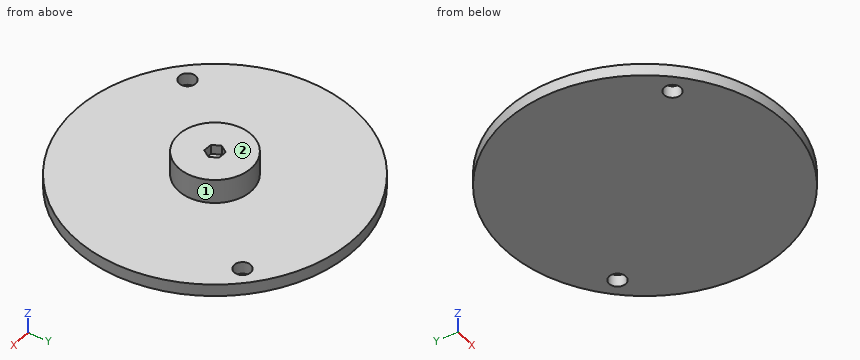
Autodesk Fusion 360 part; units mm, degrees
sketch "Sketch1" plane through (0, 0, 0) normal (0, 0, 1) x (1, 0, 0)
  circle A0 centre (0, 0) radius 18.2563
  line L0 (0, 0) -> (18.2563, 0) construction
  circle A1 centre (22.4506, 22.4506) radius 2.159
  circle A2 centre (-22.4506, -22.4506) radius 2.159
  circle A3 centre (0, 0) radius 9.525
  circle A4 centre (0, 0) radius 36.5125
  circle A5 centre (0, 0) radius 31.75
  line L1 (0, 0) -> (22.4506, 22.4506)
  line L2 (0, 0) -> (21.082, 0) construction
  line L3 (0, 0) -> (-22.4506, -22.4506)
  line L4 (0, 0) -> (21.082, 0) construction
  dimension "d1" = 36.5125
  dimension "d16" = 4.318
  dimension "d18" = 4.318
  dimension "d24" = 19.05
  dimension "d33" = 73.025
  dimension "d34" = 63.5
  dimension "d35" = 45
  dimension "d36" = 135
extrude "Extrude2" add sketch "Sketch1" along normal blind 3.175 contours A0 A3 L1 L3 | A0 A3 L1 L3 | A3 L1 L3 | A3 L1 L3
sketch "Sketch2" plane through (0, 0, 3.175) normal (0, 0, 1) x (-1, 0, 0)
  circle A0 centre (0, 0) radius 18.2563
  circle A1 centre (0, 0) radius 9.525
  dimension "d27" = 19.05
extrude "Extrude3" add sketch "Sketch2" along normal blind 6.35 contours A1
sketch "Sketch3" plane through (0, 0, 9.525) normal (0, 0, 1) x (-1, 0, 0)
  circle A0 centre (0, 0) radius 9.525
  line L0 (-1.2943, -1.9151) -> (1.0113, -2.0784)
  line L1 (1.0113, -2.0784) -> (2.3056, -0.1633)
  line L2 (2.3056, -0.1633) -> (1.2943, 1.9151)
  line L3 (1.2943, 1.9151) -> (-1.0113, 2.0784)
  line L4 (-1.0113, 2.0784) -> (-2.3056, 0.1633)
  line L5 (-2.3056, 0.1633) -> (-1.2943, -1.9151)
  dimension "d42" = 2.3114
extrude "Extrude7" add sketch "Sketch1" along normal blind 3.175 contours A0 A1 A2 A5 L1 L3 | A0 A1 A2 A5 L1 L3 | A4
extrude "Extrude8" cut sketch "Sketch3" against normal blind 2.3813 contours L0 L1 L2 L3 L4 L5
extrude "Extrude6" add sketch "Sketch1" along normal blind 3.175 contours A0 A1 A2 A5 L1 L3 | A0 A1 A2 A5 L1 L3 | A4
extrude "Extrude4" cut sketch "Sketch3" against normal blind 2.5 contours L0 L1 L2 L3 L4 L5
extrude "Extrude5" add sketch "Sketch1" along normal blind 3.175 contours A0 A1 A2 A5 L1 L3 | A0 A1 A2 A5 L1 L3 | A4
equation "d1 = ( 23 / 16 ) * 1 in"
equation "d45 = ( -3 / 32 ) * 1 in"
Source: CAD feature listing. Evaluate the final solid. Frame: model axes, mm. Face numbers are marked on the shaded views. A direction names the side the tool comes from. Round coordinates to 2 decimals unless told otherwise and drop trailing zeros. Order: outer loops, then holes, each group sorted by start corner. A loop starts at its lowest first (then second) coordinate and runs counter-clockwise, first axis right, second up. Notation, with made-up numbers: (31, 58.25) -> (48, 58.25) arc R24 ccw to (48, 78.25) -> close; hole circle Ø9 at (-31, 52). An arc over 180 degrees is marked (long way). One line per item, written item: value. Start each with the question number.
Q1. Material intervals for probe 1 along Z at (x, y) = (2.5, -24) (3 decimals); probe 2 along X at (y, z) = (1.5, 9); probe 3 along Y at (x, z) = (-30.5, 1), sorted ascending.
Q2. Section query B-B (z = 1). Return the cut outline in (x, y) (1 decimal).
Q3. Section query A-A (x = -5). Return the cut outline in (y, z) (3 decimals).
Q4. Section query C-C (y = -26). Return the cut outline in (x, z) (3 decimals).
Q5. Section query D-D (x = 3.5). Return the cut outline in (y, z) (3 decimals).
Q6. Pin query (flat end, axial travel): pin 1 (5.5 mm diameter, centred on x = 22.45, y = 22.45, fed in from +Z) (3 decimals); pin 2 (4 mm diameter, centred on y = 7.5, z = 4.5, fed in from +X); pin 3 (1.5 mm diameter, centred on x = -22, z = 4.5, fed in from +Y); pin 4 (2 mm diameter, centred on x = 0.5, y = 0.5, fed in from +Z) (3 decimals). Return the tip coordinate at first contact, or that it passes through.
Q7. Access query for the marked faces 1 and 2. Directions: +Z, -Z, +X, -X, +Y, -Y. A direction counts if a zero-diameter tool reaches every point of the face in a straight line with its end or side. Return the directions, or none.
Findings below:
1. probe 1: 0 to 3.175
1. probe 2: -9.41 to -1.4, 1.5 to 9.41
1. probe 3: -20.07 to 20.07
2. outline: circle Ø73 at (0, 0); hole circle Ø4.3 at (-22.5, -22.5); hole circle Ø4.3 at (22.5, 22.5)
3. outline: (-36.169, 0) -> (36.169, 0) -> (36.169, 3.175) -> (8.107, 3.175) -> (8.107, 9.525) -> (-8.107, 9.525) -> (-8.107, 3.175) -> (-36.169, 3.175) -> close
4. outline: (-25.635, 0) -> (25.635, 0) -> (25.635, 3.175) -> (-25.635, 3.175) -> close
5. outline: (-36.344, 0) -> (36.344, 0) -> (36.344, 3.175) -> (8.859, 3.175) -> (8.859, 9.525) -> (-8.859, 9.525) -> (-8.859, 3.175) -> (-36.344, 3.175) -> close
6. pin 1: z = 3.175
6. pin 2: x = 36.02
6. pin 3: through
6. pin 4: z = 7.025
7. face 1: +Z
7. face 2: +Z, +X, -X, +Y, -Y
